Geometry check sheet. Reference: drawing and pictorial views, mm from the part's lowest x, y, z. A direction names the side the tool comes from. Give positions to 0.01 mm unless a question says otherwise; leave off trailing zeros. Write each loop counter-clockwise with the first axis right and the second up, starting at its lowest first coordinate (ties: lowest second). Pieces come first, ordered by that corner, then holes. Notation, with made-up numbers: (-18.5, 17) -> (-7.5, 17) arc R31 ccw to (-7.5, 46) -> close; hole circle Ø9 at (-19, -26.75). An arc over 180 degrees is marked (long way). Use a Markdown table: item, result. Add a question column.
1. Scan lines: probe 1 along Y at (x, z) = (114, 22); probe 2 along Z at (x, y) = (74.5, 25); probe 3 along X at (y, z) = (33.5, 125.5). Record each from-to range of solid material in increasing order. Write a range as [from, to].
2. Cross-section at B-B (z = 76.2). Enter the section's corners in (x, y).
3. Set-up check for the marked faces 1 and 2: record each of +Z, -Z, +X, -X, +Y, -Y from which the full face is reachable in a straight line by a thin tool's end or side.
4. Cross-section at D-D (z = 18). Enter the section's corners in (x, y).
5. Cross-section at A-A (x = 76.2). Enter the section's corners in (y, z).
6. Gauge pin test, flat ends, axial feed: P1, Ø12, axis at x = 54, y = 9.5, coming from the +Z side; P2, Ø3, axis at x = 29, y = 20, coming from the -Z side (3 decimals); P3, Ø10, axis at y = 17.5, z = 107.5, coming from the +X side. Record the tip position at first contact, or that the pin passes through.
7. Cross-section at C-C (y = 30.5). Enter the section's corners in (x, z), then the cut area to 3 significant figures.
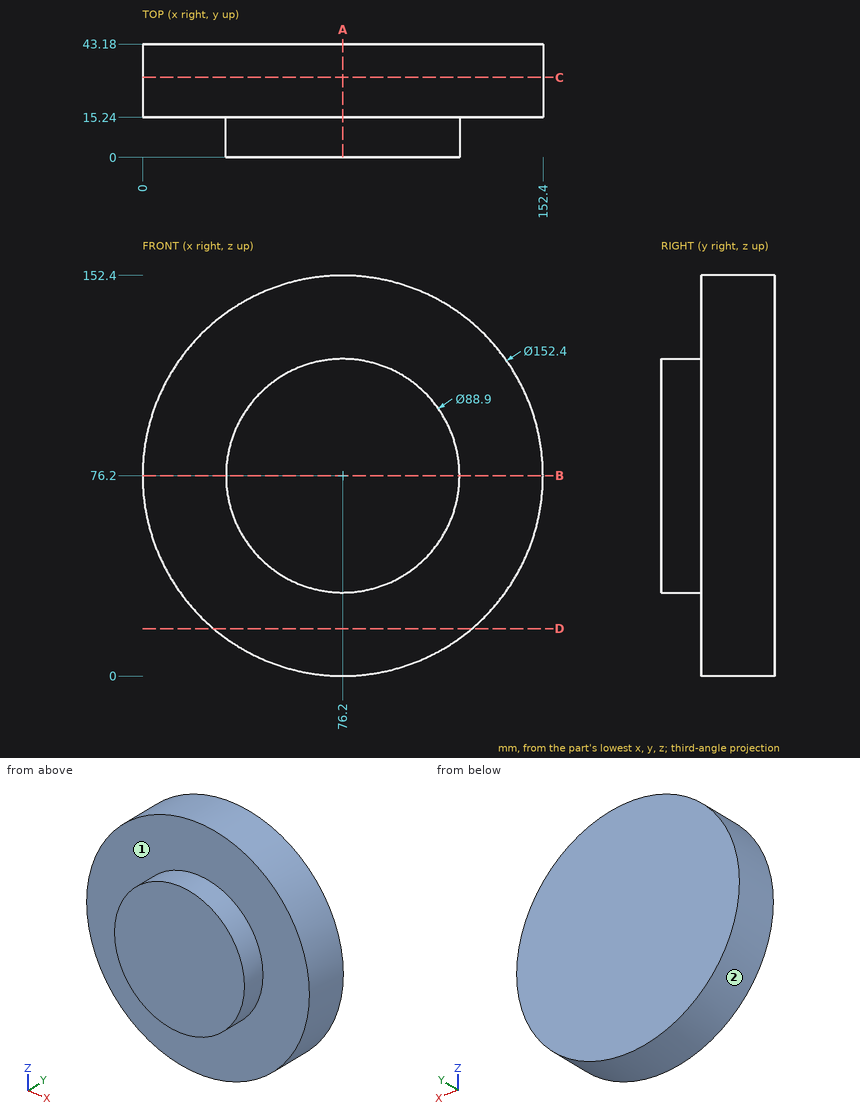
Worked answers:
| question | item | result |
|---|---|---|
| 1 | probe 1 | y = [15.24, 43.18] |
| 1 | probe 2 | z = [0.02, 152.38] |
| 1 | probe 3 | x = [18.1, 134.3] |
| 2 | outline | (0, 15.24) -> (31.75, 15.24) -> (31.75, 0) -> (120.65, 0) -> (120.65, 15.24) -> (152.4, 15.24) -> (152.4, 43.18) -> (0, 43.18) -> close |
| 3 | face 1 | -Y |
| 3 | face 2 | +Y, -Y |
| 4 | outline | (27.01, 15.24) -> (125.39, 15.24) -> (125.39, 43.18) -> (27.01, 43.18) -> close |
| 5 | outline | (0, 31.75) -> (15.24, 31.75) -> (15.24, 0) -> (43.18, 0) -> (43.18, 152.4) -> (15.24, 152.4) -> (15.24, 120.65) -> (0, 120.65) -> close |
| 6 | P1 | stops at z = 149.6 |
| 6 | P2 | stops at z = 15.225 |
| 6 | P3 | stops at x = 147.72 |
| 7 | outline | circle Ø152.4 at (76.2, 76.2) |
| 7 | area | 18,200 mm² |
